Check sheet for the modelled part. Datum: model origin and axes. Units: mm. A direction names the side the tool comes from. Round coordinates to 2 decimals unless told otherwise and drop trailing zeros. Loops run counter-clockwise (first coordinate to the right, second up) from the corner with the lowest first, then second, coordinate; pieces in that order, holes last. Notation, with made-up numbers: (-7, 56.25) -> (29, 56.25) arc R24 ccw to (29, 73.25) -> close; hole circle Ø3 at (30.5, 4.25). An arc over 180 degrees is marked (long way). One line per question, with ' | ' between items.
```python
from build123d import *

# Parameters (mm, degrees)
SKETCH_1_W               = 50
SKETCH_1_H               = 50
EXTRUDE_1_DEPTH          = 70
SKETCH_2_R               = 40
EXTRUDE_2_DEPTH          = 100
SKETCH_3_R               = 21
EXTRUDE_3_DEPTH          = 70
SKETCH_5_R               = 15
CUT_EXTRUDE_1_DEPTH      = 252.843205189
CUT_EXTRUDE_2_DEPTH      = 50
CUT_EXTRUDE_2_DEPTH_BACK = 50
SKETCH_6_R               = 12.5
CUT_EXTRUDE_START        = -8
CUT_EXTRUDE_3_DEPTH      = 239.576560151
SKETCH_10_W              = 4
SKETCH_10_H              = 3
FILLET_1_R               = 2


with BuildPart() as part:
    # Sketch 1 → Extrude 1 (new body)
    with BuildSketch(Plane.XY):
        Rectangle(SKETCH_1_W, SKETCH_1_H)
    extrude(amount=EXTRUDE_1_DEPTH)

    # Sketch 2 → Extrude 2 (add)
    with BuildSketch(Plane.XY.offset(70)):
        Circle(SKETCH_2_R)
    extrude(amount=EXTRUDE_2_DEPTH)

    # Sketch 3 → Extrude 3 (add)
    with BuildSketch(Plane.XY.offset(170)):
        Circle(SKETCH_3_R)
    extrude(amount=EXTRUDE_3_DEPTH)

    # Sketch 5 → Cut-Extrude 1 (cut, through all)
    with BuildSketch(Plane.XZ.offset(25)):
        with Locations(Location((0, 35, 0), (0, 0, 270))):
            Circle(SKETCH_5_R)
    extrude(amount=-CUT_EXTRUDE_1_DEPTH, mode=Mode.SUBTRACT)

    # Sketch 6 → Cut-Extrude 2 (cut, two sides: drawn at the far end of the back side and taken through both)
    with BuildSketch(Plane(origin=(0, 0, 0), x_dir=(1, 0, 0), z_dir=(0, 1, 0)).offset(-CUT_EXTRUDE_2_DEPTH_BACK)):
        with Locations(Location((0, -120, 0), (0, 0, 90))):
            Circle(SKETCH_6_R)
    extrude(amount=CUT_EXTRUDE_2_DEPTH + CUT_EXTRUDE_2_DEPTH_BACK, mode=Mode.SUBTRACT)

    # Sketch 7 → Cut-Revolve 1 (revolve, cut)
    with BuildSketch(Plane(origin=(0, 0, 0), x_dir=(1, 0, 0), z_dir=(0, 1, 0)), mode=Mode.PRIVATE) as cut_revolve_1_sk:
        Polygon((-40, -120), (-40, -112), (-22, -112), (-17.381197846, -120), align=None)
    revolve(cut_revolve_1_sk.sketch.rotate(Axis((-40, 0, 120), (1, 0, 0)), 180), axis=Axis((-40, 0, 120), (1, 0, 0)), mode=Mode.SUBTRACT)

    # Sketch 8 → Cut-Extrude 3 (cut, through all)
    with BuildSketch(Plane(origin=(0, 0, 0), x_dir=(0, 0, -1), z_dir=(1, 0, 0)).offset(CUT_EXTRUDE_START)):
        with BuildLine():
            Line((-228, 5), (-206, 5))
            ThreePointArc((-206, 5), (-201, 0), (-206, -5))
            Line((-206, -5), (-228, -5))
            ThreePointArc((-228, -5), (-233, 0), (-228, 5))
        make_face()
    extrude(amount=-CUT_EXTRUDE_3_DEPTH, mode=Mode.SUBTRACT)

    # Sketch 10 → Cut-Revolve 2 (revolve, cut)
    with BuildSketch(Plane(origin=(0, 0, 0), x_dir=(1, 0, 0), z_dir=(0, 1, 0)), mode=Mode.PRIVATE) as cut_revolve_2_sk:
        with Locations((-19, -171.5)):
            Rectangle(SKETCH_10_W, SKETCH_10_H)
    revolve(cut_revolve_2_sk.sketch.rotate(Axis((0, 0, 240), (0, 0, -1)), 180), axis=Axis((0, 0, 240), (0, 0, -1)), mode=Mode.SUBTRACT)

    # Fillet 1
    fillet_1_edges = [part.edges().sort_by_distance(p)[0] for p in [
        (-17, 0, 170),
    ]]
    fillet(fillet_1_edges, radius=FILLET_1_R)


solid = part.part
```
(1) Go/stop test with flat-tipped pins: pin 1 (2 mm diameter, centred on y = 23.5, z = 180.5, fed in from -X); pin 2 (1.5 mm diameter, centred on y = 4.5, z = 212.5, fed in from +X); pin 3 (4 mm diameter, centred on y = -16.5, z = 164, fed in from -X); pin 4 (5 mm diameter, centred on y = 0.5, z = 225, fed in from -X). Record where each tip stops, or that it passes through.
Answer:
pin 1: passes through | pin 2: stops at x = 20.66 | pin 3: stops at x = -37.28 | pin 4: stops at x = -8
(2) Mould release check, pull along Y, two halves, no side actions. Record for faces 5 (the face through (0, 25, 19)), 6 (the face through (-30.87, -2.4, 127.63)), 7 (the face through (0.66, -0.35, 49.985)), 8 (the face through (-18.12, -0.38, 121.22)): +Y half, -Y half, draft (parallel to the pull), parting line (faces both ways), or undercut.
Answer:
face 5: +Y half | face 6: undercut | face 7: draft | face 8: undercut
(3) Sectioned sample at C-C, the plane y = 29.5. Record the cut outline in (x, z).
Answer:
outline: (-27.01, 70) -> (27.01, 70) -> (27.01, 170) -> (-27.01, 170) -> close; hole circle Ø25 at (0, 120)
(4) Sectioned sample at B-B, the plane z = 35. Record the cut outline in (x, y).
Answer:
outline: (-25, -25) -> (-15, -25) -> (-15, 25) -> (-25, 25) -> close; (15, -25) -> (25, -25) -> (25, 25) -> (15, 25) -> close
(5) Scan lines: probe 1 along X at (y, z) = (1, 36); probe 2 along Z at (x, y) = (2, 15.5); probe 3 along Z at (x, y) = (27.5, -5.5). Record each from-to range of solid material in increasing order.
Answer:
probe 1: x = -25 to -14.97, 14.97 to 25 | probe 2: z = 0 to 20.13, 49.87 to 107.66, 132.34 to 240 | probe 3: z = 70 to 170
(6) Sectioned sample at A-A, the plane x = 0. Record the cut outline in (y, z).
Answer:
outline: (-40, 70) -> (-25, 70) -> (-25, 50) -> (25, 50) -> (25, 70) -> (40, 70) -> (40, 107.5) -> (-40, 107.5) -> close; (-40, 132.5) -> (40, 132.5) -> (40, 170) -> (19, 170) arc R2 cw to (17, 172) -> (17, 173) -> (21, 173) -> (21, 240) -> (-21, 240) -> (-21, 173) -> (-17, 173) -> (-17, 172) arc R2 cw to (-19, 170) -> (-40, 170) -> close; (-25, 0) -> (25, 0) -> (25, 20) -> (-25, 20) -> close
(7) Set-up check for faces 1 (the face through (25, 0, 35)), 2 (the face through (0, -25, 19)), 3 (the face through (-14, 0, 233)), 4 (the face through (7.7, 15.5, 173)): record each of +Z, -Z, +X, -X, +Y, -Y from which the full face is reachable in a straight line by a thin tool's end or side.
Answer:
face 1: -Z, +X, +Y, -Y | face 2: -Z, +X, -X, -Y | face 3: -X | face 4: none
(8) Sectioned sample at D-D, the plane z = 94. Record the cut outline in (x, y), and give its area (3 significant figures).
Answer:
outline: circle Ø80 at (0, 0) | area: 5,030 mm2
